Verification items for the finished model (mm, model axes). Face numbers are marked on the shaded views. Round coordinates to 2 decimals unless told otherwise and drop trailing zeros. Write each loop counter-clockwise with the first axis right and the second up, starting at its lowest first coordinate (ties: lowest second). Pieces come first, ordered by that corner, then holes.
from build123d import *

# Parameters (mm, degrees)
SKETCH_1_W          = 250
SKETCH_1_H          = 20
SKETCH_1_W_2        = 60
SKETCH_1_H_2        = 12
EXTRUDE_1_DEPTH     = 4
SKETCH_2_W          = 20
SKETCH_2_H          = 140
SKETCH_2_R          = 1.6
EXTRUDE_2_DEPTH     = 5
SKETCH_3_W          = 64
SKETCH_3_H          = 15
SKETCH_3_R          = 1.1
EXTRUDE_3_DEPTH     = 4
SKETCH_4_W          = 49.65332139
SKETCH_4_H          = 44.815301216
CUT_EXTRUDE_1_DEPTH = 4


with BuildPart() as part:
    # 草图1 → 凸台-拉伸1 (new body)
    with BuildSketch(Plane(origin=(0, 0, 0), x_dir=(1, 0, 0), z_dir=(0, 1, 0))):
        Rectangle(SKETCH_1_W, SKETCH_1_H)
        Rectangle(SKETCH_1_W_2, SKETCH_1_H_2, mode=Mode.SUBTRACT)
    extrude(amount=EXTRUDE_1_DEPTH)

    # 草图2 → 凸台-拉伸2 (add)
    with BuildSketch(Plane.ZY.offset(125)):
        with Locations((0, 70)):
            Rectangle(SKETCH_2_W, SKETCH_2_H)
        with Locations((-5, 135)):
            Circle(SKETCH_2_R, mode=Mode.SUBTRACT)
        with Locations(Location((5, 135, 0), (0, 0, 180))):
            Circle(SKETCH_2_R, mode=Mode.SUBTRACT)
    extrude_2 = extrude(amount=-EXTRUDE_2_DEPTH)

    # 镜向1: 凸台-拉伸2 across plane
    add(extrude_2.mirror(Plane(origin=(0, 0, 0), x_dir=(0, 0, 1), z_dir=(1, 0, 0))))

    # 草图3 → 凸台-拉伸3 (add)
    # profile 1 of 2: a face of its own
    with BuildSketch(Plane(origin=(0, 4, 0), x_dir=(1, 0, 0), z_dir=(0, 1, 0))):
        with Locations((0, 17.5)):
            Rectangle(SKETCH_3_W, SKETCH_3_H)
        with Locations(Location((-28, 21, 0), (0, 0, 270))):
            Circle(SKETCH_3_R, mode=Mode.SUBTRACT)
        with Locations(Location((28, 21, 0), (0, 0, 270))):
            Circle(SKETCH_3_R, mode=Mode.SUBTRACT)
    # profile 2 of 2: a face of its own
    with BuildSketch(Plane(origin=(0, 4, 0), x_dir=(1, 0, 0), z_dir=(0, 1, 0))):
        with Locations((0, -17.5)):
            Rectangle(SKETCH_3_W, SKETCH_3_H)
        with Locations(Location((-28, -21, 0), (0, 0, 270))):
            Circle(SKETCH_3_R, mode=Mode.SUBTRACT)
        with Locations(Location((28, -21, 0), (0, 0, 270))):
            Circle(SKETCH_3_R, mode=Mode.SUBTRACT)
    extrude(amount=-EXTRUDE_3_DEPTH)

    # 草图4 → 切除-拉伸1 (cut)
    with BuildSketch(Plane(origin=(0, 4, 0), x_dir=(1, 0, 0), z_dir=(0, 1, 0))):
        Rectangle(SKETCH_4_W, SKETCH_4_H)
    extrude(amount=-CUT_EXTRUDE_1_DEPTH, mode=Mode.SUBTRACT)


solid = part.part
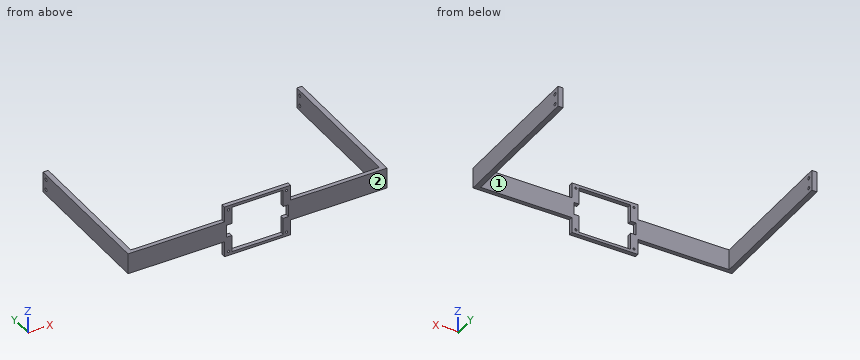
Q1. Sectioned sample at B-B (x = 10). Enter the section's corners in (y, z).
Recorded:
outline: (0, -25) - (4, -25) - (4, -22.41) - (0, -22.41) - close; (0, 22.41) - (4, 22.41) - (4, 25) - (0, 25) - close
Q2. Depth check by flat-ended pin: P1, Ø1.2, axis at y = 3, z = 16, coming from the -X side; P2, Ø6, axis at x = 58.5, z = 11, coming from the +Y side; P3, Ø1.2, axis at y = 1.5, z = 13.5, coming from the +X side. Enter the tip coordinate at first touch or a pass-through.
Recorded:
P1: stops at x = -32
P2: stops at y = 4
P3: stops at x = 32
Q3. Sectioned sample at A-A (z = -0.5). Enter the section's corners in (x, y).
Recorded:
outline: (-125, 0) - (-30, 0) - (-30, 4) - (-120, 4) - (-120, 140) - (-125, 140) - close; (30, 0) - (125, 0) - (125, 140) - (120, 140) - (120, 4) - (30, 4) - close
Q4. Material ranges on line 1 along X through (y, z) = (2, -21); line 2 along Y through (x, z) = (-122, 5); line 3 along Z through (x, y) = (-122, 135), recorded low to high.
Recorded:
line 1: x = -32 to -29.1, -26.9 to -24.83, 24.83 to 26.9, 29.1 to 32
line 2: y = 0 to 133.4, 136.6 to 140
line 3: z = -10 to -6.6, -3.4 to 3.4, 6.6 to 10
Q5. Sectioned sample at D-D (x = 75.5). Enter the section's corners in (y, z), plus the area to 3 significant figures.
Recorded:
outline: (0, -10) - (4, -10) - (4, 10) - (0, 10) - close
area: 80.0 mm2
Q6. Release check for a two-part mould opening along X. For the marked faces 1 and 2 record: released by +X, released by -X, zero draft, split by the parting line, or undercut.
Recorded:
face 1: undercut
face 2: zero draft
Q7. Sectioned sample at C-C (y = 33). Enter the section's corners in (x, z), plus the area to 3 significant figures.
Recorded:
outline: (-125, -10) - (-120, -10) - (-120, 10) - (-125, 10) - close; (120, -10) - (125, -10) - (125, 10) - (120, 10) - close
area: 200 mm2
